Input: part model. Units: mm. Frame: model coordinates. A direction names the side the tool comes from. Round coordinates to 2 decimals unless told otherwise and drop trailing zeros. Loops run counter-clockwise (first coordinate to the right, second up) from the corner with the lowest first, then second, coordinate; pieces in that order, holes last.
(1) Draft query along Y for faces 4 (the face through (-9, -3, -15)), 5 (the face through (-7, -11, -51.8)), 6 (the face through (-7.655, 2.465, -12.216)). Return one class per face: released by +Y, released by -Y, zero draft, split by the parting line, or undercut.
(2) Cut plane B-B, the plane z = -55. Output: boundary loops of the cut face in (x, y).
(3) Cut plane D-D, the plane z = -31. Output: boundary loops of the cut face in (x, y), and give its area (3 significant figures).
(4) First-contact query: pin 1 Ø3 at (x, y) = (-8.5, -11.5) entering from -Z; pin 2 Ø2.5 at (x, z) = (-5.5, -32.5) entering from +Y; pin 3 Ø5.5 at (x, z) = (-5.7, -11.6) entering from -Y. Flat tips, straight axial feed; report the tip coordinate or a pass-through.
(5) Line query: line 1 (Z direction, x = -5.7, y = 3.45); line 2 (Z direction, x = -5.7, y = -1); line 3 (X direction, y = 5.25, z = -43). Output: solid intervals per line, ascending.
(6) Cut plane C-C, the plane x = -4.5. Give the number of separate pieces and of enclosed holes in the cut face, and give its area (3 significant figures).
(7) Access query for faces 1 (the face through (-2.803, -1.479, -13.821)), 2 (the face through (-6.431, -14.977, -49.335)), 3 (the face through (-7, -16, -46.8)). Directions: +Z, -Z, +X, -X, +Y, -Y. A direction counts if a zero-diameter tool reaches every point of the face in a straight line with its end or side. Return the directions, or none.
(8) Cut plane A-A, the plane z = -11.6. Output: boundary loops of the cut face in (x, y).
Autodesk Inventor part; units mm, degrees
ref_plane "Work Plane1" through (-1.6, -3, -51.8) normal (0, 0, 1) x (1, 0, 0)
ref_plane "Work Plane2" through (-11.4, -8.0259, -51.8) normal (-0.9659, -0.2588, 0) x (0.2588, -0.9659, 0)
ref_plane "YZ Plane" through (0, 0, 0) normal (1, 0, 0) x (0, 1, 0)
sketch "Sketch1" plane through (0, 0, 0) normal (0, 1, 0) x (-1, 0, 0)
  line L0 (0, 0) -> (11.4, 0) construction
  line L1 (11.4, 0) -> (11.4, -64.7) construction
  line L2 (11.4, -64.7) -> (0, -64.7) construction
  line L3 (0, -64.7) -> (0, 0) construction
  line L4 (5.7, 0) -> (5.7, -64.7) construction
  line L5 (11.4, -32.35) -> (0, -32.35) construction
  circle A0 centre (5.7, -11.6) radius 1.6 construction
  circle A1 centre (5.7, -11.6) radius 2.05
  circle A2 centre (5.7, -21.3) radius 1.6 construction
  circle A3 centre (5.7, -21.3) radius 2.05 construction
  circle A4 centre (5.7, -31) radius 1.6 construction
  circle A5 centre (5.7, -31) radius 2.05 construction
  circle A6 centre (5.7, -40.7) radius 1.6 construction
  circle A7 centre (5.7, -40.7) radius 2.05 construction
  circle A8 centre (5.7, -50.4) radius 1.6 construction
  circle A9 centre (5.7, -50.4) radius 2.05 construction
  circle A10 centre (5.7, -60.1) radius 1.6 construction
  circle A11 centre (5.7, -60.1) radius 2.05
  line L6 (8.2, 0) -> (3.2, 0) construction
  line L7 (3.2, 0) -> (3.2, -64.7)
  line L8 (3.2, -64.7) -> (8.2, -64.7) construction
  line L9 (8.2, -64.7) -> (8.2, 0)
  circle A12 centre (5.7, -11.6) radius 2.5 construction
  circle A13 centre (5.7, -5.7) radius 5.7 construction
  circle A14 centre (8.2, -61.5) radius 3.2 construction
  line L10 (0, -64.7) -> (3.2, -64.7) construction
  line L11 (1.6, -64.7) -> (1.6, 0)
  circle A15 centre (5.7, -60.1) radius 3.65
  circle A16 centre (5.7, -50.4) radius 3.65 construction
  circle A17 centre (5.7, -40.7) radius 3.65 construction
  circle A18 centre (5.7, -31) radius 3.65 construction
  circle A19 centre (5.7, -21.3) radius 3.65 construction
  circle A20 centre (5.7, -11.6) radius 3.65
  arc A21 (8.2, -64.7) -> (11.4, -61.5) centre (8.2, -61.5) ccw
  arc A22 (11.4, -5.7) -> (5.7, 0) centre (5.7, -5.7) ccw
  line L12 (11.4, -61.5) -> (11.4, -5.7)
  line L13 (1.6, -64.7) -> (8.2, -64.7)
  line L14 (1.6, 0) -> (5.7, 0)
  point P0 (5.7, -10)
  point P1 (5.7, -61.7)
  point P2 (8.2, -0.5775)
  dimension "d0" = 3.2
  dimension "d1" = 4.1
  dimension "d4" = 9.7
  dimension "d9" = 6.5
  dimension "d10" = 10
  dimension "d11" = 3
  dimension "d12" = 0.9
  dimension "d13" = 3.2
  dimension "d14" = 7.3
  dimension "d39" = 48.5
extrude "Extrusion1" add sketch "Sketch1" along normal blind 6 contours L7 A20 A15 L13 L11 L14 | L7 A20 | A20 L9 | L9 A22 L12 A21 A15 A20 | L7 A15 | A15 L9
extrude "Extrusion3" add sketch "Sketch1" along normal blind 5 contours L14 A22 L9 A20 L7 | A20 L9 L7 | A20 L9 A15 L7 | A15 L9 L7 | L7 A15 L9 L13
extrude "Extrusion2" add sketch "Sketch1" against normal blind 3 contours L14 A22 L9 A20 L7 | L7 A20 A15 L13 L11 L14 | A20 L9 A15 L7 | L9 A22 L12 A21 A15 A20 | L7 A15 L9 L13
sketch "Sketch2" plane through (0, -3, 0) normal (0, -1, 0) x (1, 0, 0)
  line L0 (-1.6, -64.7) -> (-1.6, 0) construction
  circle A0 centre (-5.7, -11.6) radius 3.65 construction
  circle A1 centre (-5.7, -60.1) radius 3.65 construction
  line L1 (-11.4, -5.7) -> (-11.4, -61.5) construction
  arc A2 (-11.4, -61.5) -> (-8.2, -64.7) centre (-8.2, -61.5) ccw construction
  line L2 (-8.2, -64.7) -> (-1.6, -64.7) construction
  arc A3 (-5.7, 0) -> (-11.4, -5.7) centre (-5.7, -5.7) ccw construction
  line L3 (-1.6, 0) -> (-5.7, 0) construction
  line L4 (-5.7, -60.1) -> (-5.7, -11.6) construction
  circle A4 centre (-5.7, -55.25) radius 4.85 construction
  circle A5 centre (-5.7, -45.55) radius 4.85 construction
  circle A6 centre (-5.7, -35.85) radius 4.85 construction
  circle A7 centre (-5.7, -26.15) radius 4.85 construction
  circle A8 centre (-5.7, -16.45) radius 4.85 construction
  line L5 (0, -51.8) -> (-11.4, -51.8) construction
  line L6 (-11.4, -51.8) -> (-11.4, -29.6) construction
  line L7 (-11.4, -29.6) -> (0, -29.6) construction
  line L8 (0, -29.6) -> (0, -51.8) construction
  line L9 (0, -51.8) -> (-11.4, -29.6) construction
  line L10 (-11.4, -51.8) -> (0, -29.6) construction
  line L11 (0, -27.1) -> (-11.4, -27.1) construction
  line L12 (-11.4, -27.1) -> (-11.4, -54.3) construction
  line L13 (-11.4, -54.3) -> (0, -54.3) construction
  line L14 (0, -54.3) -> (0, -27.1) construction
  line L15 (0, -27.1) -> (-11.4, -54.3) construction
  line L16 (-11.4, -27.1) -> (0, -54.3) construction
  line L17 (-11.4, -54.3) -> (-1.6, -54.3)
  line L18 (-1.6, -54.3) -> (-1.6, -51.8)
  line L19 (-1.6, -51.8) -> (-11.4, -51.8)
  line L20 (-11.4, -51.8) -> (-11.4, -54.3)
  point P0 (0, 0)
  point P1 (-5.7, -50.4)
  point P2 (-5.7, -40.7)
  point P3 (-5.7, -31)
  point P4 (-5.7, -21.3)
  dimension "d21" = 22.2
  dimension "d22" = 2.5
ref_plane "Work Plane1" through (-1.6, -3, -51.8) normal (0, 0, 1) x (1, 0, 0)
sketch "Sketch3" plane through (-1.6, -3, -51.8) normal (0, 0, 1) x (1, 0, 0)
  line L0 (0, 0) -> (-9.8, 0)
  line L1 (0, 0) -> (0, -2.4)
  line L2 (0, -2.4) -> (-9.8, -5.0259)
  line L3 (-9.8, -5.0259) -> (-9.8, 0)
  line L4 (0, -2.4) -> (-9.8, -2.4) construction
  line L5 (0, -2.4) -> (0, -10.6822)
  line L6 (0, -10.6822) -> (-9.8, -13.3081)
  line L7 (-9.8, -13.3081) -> (-9.8, -5.0259)
  line L8 (-9.8, -13.3081) -> (-9.8, -15.3081)
  line L9 (-9.8, -15.3081) -> (0, -12.6822)
  line L10 (0, -12.6822) -> (0, -10.6822)
  line L11 (-9.8, -5.0259) -> (-7.7294, -12.7533) construction
  point P0 (1.6, 3)
  dimension "d23" = 2.4
  dimension "d24" = 15
  dimension "d25" = 9.8
  dimension "d26" = 2
  dimension "d27" = 8
extrude "Extrusion4" add sketch "Sketch3" against normal blind 2
extrude "Extrusion5" add sketch "Sketch3" along normal blind 22.2 contours L1 L2 L3 L0
ref_plane "Work Plane2" through (-11.4, -8.0259, -51.8) normal (-0.9659, -0.2588, 0) x (0.2588, -0.9659, 0)
sketch "Sketch4" plane through (-11.4, -8.0259, -51.8) normal (-0.9659, -0.2588, 0) x (0.2588, -0.9659, 0)
  line L0 (0, 0) -> (0, 22.2)
  arc A0 (0, 22.2) -> (0, 0) centre (24.4688, 11.1) ccw
  line L1 (-2.4, 11.1) -> (-2.4273, 22.2)
  line L2 (-4.8546, 22.2) -> (0, 22.2)
  line L3 (0, 22.2) -> (-2.4273, 22.2)
  point P0 (-4.8019, 51.8)
  point P1 (0, 11.1)
  dimension "d32" = 2.4
extrude "Extrusion6" cut sketch "Sketch4" against normal through all
extrude "Extrusion7" add sketch "Sketch3" along normal blind 5 contours L10 L9 L8 L6
properties part number "Right-Brush-Bottom"
Reported:
1. face 4: released by -Y
1. face 5: undercut
1. face 6: zero draft
2. outline: (-11.4, -3) - (-1.6, -3) - (-1.6, 6) - (-3.2, 6) - (-3.2, 5) - (-8.2, 5) - (-8.2, 6) - (-11.4, 6) - close
3. outline: (-11.4, -5.52) - (-1.6, -2.89) - (-1.6, 6) - (-3.2, 6) - (-3.2, 5) - (-8.2, 5) - (-8.2, 6) - (-11.4, 6) - close
3. area: 95.0 mm2
4. pin 1: stops at z = -53.8
4. pin 2: stops at y = 5
4. pin 3: stops at y = 0
5. line 1: z = -64.7 to -62.15, -58.05 to -13.65, -9.55 to 0
5. line 2: z = -64.7 to -63.75, -56.45 to -15.25, -7.95 to 0
5. line 3: x = -11.4 to -8.2, -3.2 to -1.6
6. separate pieces: 3
6. enclosed holes: 0
6. area: 504 mm2
7. face 1: -Y
7. face 2: +Z, -X
7. face 3: +Z, +X, -X, -Y
8. outline: (-11.4, -3) - (-9.35, -3) - (-9.35, 0) - (-7.75, 0) - (-7.75, 5) - (-8.2, 5) - (-8.2, 6) - (-11.4, 6) - close; (-3.65, 0) - (-2.05, 0) - (-2.05, -3) - (-1.6, -3) - (-1.6, 6) - (-3.2, 6) - (-3.2, 5) - (-3.65, 5) - close
